Check sheet for the modelled part. Datum: model origin and axes. Units: mm. Face numbers are marked on the shaded views. A direction names the side the tool comes from. Give positions to 0.01 mm unless a question says otherwise; leave off trailing zeros. Order: outer loops, then holes, each group sorted by start corner. A loop starts at its lowest first (then second) coordinate and runs counter-clockwise, first axis right, second up.
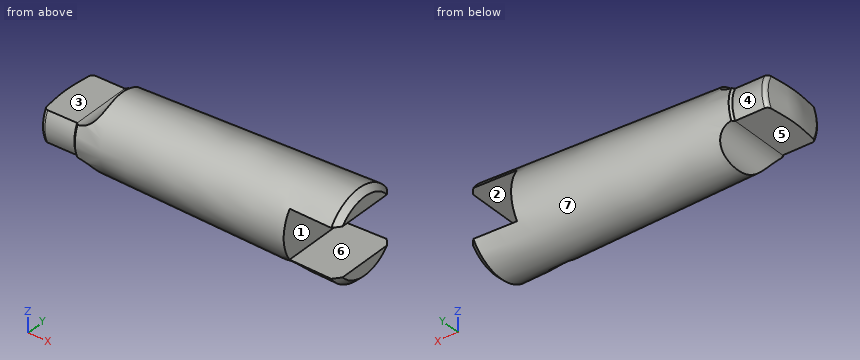
Autodesk Inventor part; units mm, degrees
ref_plane "YZ Plane" through (0, 0, 0) normal (1, 0, 0) x (0, 1, 0)
ref_plane "XZ Plane" through (0, 0, 0) normal (0, 1, 0) x (-1, 0, 0)
ref_plane "XY Plane" through (0, 0, 0) normal (0, 0, 1) x (1, 0, 0)
sketch "Sketch1" plane through (0, 0, 0) normal (0, 0, 1) x (1, 0, 0)
  line L0 (0, 0) -> (0, 18.2735) construction
  line L1 (0, 18.2735) -> (20.5646, 18.8146) construction
  line L2 (155.5, 22.3653) -> (155.5, 0)
  line L3 (155.5, 0) -> (0, 0)
  line L4 (149.2, 22.1995) -> (149.2, 0) construction
  line L5 (0, 0) -> (2.3398, 16.0387)
  line L6 (4.3188, 17.75) -> (19.5, 17.75)
  line L7 (19.5, 17.75) -> (20.5646, 18.8146)
  arc A0 (4.3188, 17.75) -> (2.3398, 16.0387) centre (4.3188, 15.75) ccw
  line L8 (20.5646, 18.8146) -> (155.5, 22.3653)
  dimension "d0" = 36.547
  dimension "d1" = 155.5
  dimension "d2" = 44.399
  dimension "d3" = 149.2
  dimension "d4" = 35.5
  dimension "d5" = 45
  dimension "d6" = 19.5
  dimension "d7" = 2
  dimension "d8" = 8.3
revolve "Revolution1" add sketch "Sketch1" angle 360 about axis through (155.5, 0, 0) along (-1, 0, 0)
sketch "Sketch2" plane through (0, 0, 0) normal (0, 1, 0) x (-1, 0, 0)
  line L0 (0, 7.95) -> (-19.5007, 7.95)
  arc A0 (-24.5298, 28.7331) -> (-19.5007, 7.95) centre (-19.5007, 18.95) ccw
  line L1 (-24.5298, 28.7331) -> (0, 28.7331)
  line L2 (0, 28.7331) -> (0, 7.95)
  line L3 (31.1, 0) -> (-186.6, 0)
  line L4 (-20.5646, 18.8146) -> (-155.5, 22.3653) construction
  point P0 (0, 0)
  point P1 (-30.5, 19.0761)
  dimension "d10" = 15.9
  dimension "d11" = 11
  dimension "d12" = 30.5
extrude "Extrusion1" cut sketch "Sketch2" along normal through all both and the other way through all
mirror "Mirror1" about plane through (0, 0, 0) normal (0, 0, 1) of "Extrusion1"
chamfer "Chamfer1" distance 3 angle 45 1 edges at (155.5, -22.3653, 0)
sketch "Sketch3" plane through (0, 0, 0) normal (0, 1, 0) x (-1, 0, 0)
  line L0 (-155.5, 12.5) -> (-130.5, 12.5)
  line L1 (-130.5, 12.5) -> (-130.5, -12.5)
  line L2 (-130.5, -12.5) -> (-155.5, -12.5)
  line L3 (-155.5, -12.5) -> (-155.5, 12.5)
  line L4 (-155.5, -19.3653) -> (-155.5, 19.3653) construction
  point P0 (0, 0)
  point P1 (-155.5, 0)
  dimension "d18" = 25
  dimension "d19" = 25
extrude "Extrusion2" cut sketch "Sketch3" along normal through all both and the other way through all
properties part number "Part005.Morse 5 shaft" material "Steel, Alloy"
(1) Release check for a two-part mould opening along Z. For the marked faces 1, 2, 3 and 4 record: released by +Z, released by -Z, zero draft, split by the parting line, or undercut.
(2) Sectioned sample at B-B (x = 23.5). Enter the section's corners in (y, z).
(3) Go/stop test with flat-tipped pins: P1, Ø12.5, axis at y = -8.5, z = -1.5, coming from the +X side; P2, Ø5.5, axis at x = 12, y = -7.5, coming from the +Z side; P3, Ø7.5, axis at x = 139, y = 0, coming from the +Z side. Record where each tip stops, or that it passes through.
(4) Thickness scan on L1, parallel to Z at x = 142, y = -13; L2, parallel to Z at x = 140.5, y = 3.5; L3, parallel to Z at x = 43.5, y = 1. Record the ranges inside material, lowest first.
(5) Tool access check on the marked faces 5, 6 and 7. Record the directions out of +Z, -Z, +X, -X, +Y, -Y that give a thin tool (end or side, any length) a straight path to the whole face; none if there is none.
(6) Sectioned sample at A-A (x = 64.5). Enter the section's corners in (y, z), plus the area to 3 significant figures.
Values follow:
1. face 1: undercut
1. face 2: undercut
1. face 3: released by +Z
1. face 4: split by the parting line
2. outline: (-16.77, -8.7) - (16.77, -8.7) arc R18.89 ccw to (16.77, 8.7) - (-16.77, 8.7) arc R18.89 ccw to start
3. P1: stops at x = 130.5
3. P2: stops at z = 7.95
3. P3: stops at z = 22.03
4. L1: z = -17.76 to -12.5, 12.5 to 17.76
4. L2: z = -21.69 to -12.5, 12.5 to 21.69
4. L3: z = -19.39 to 19.39
5. face 5: -Z, -X, +Y, -Y
5. face 6: +X, +Y, -Y
5. face 7: -X
6. outline: circle Ø39.94 at (0, 0)
6. area: 1,250 mm2
